```python
from build123d import *

# Parameters (mm, degrees)
SKETCH3_W                    = 914.4
SKETCH3_H                    = 609.6
BOSS_EXTRUDE1_DEPTH          = 0.79375
SKETCH4_OUTSIDE_W            = 1136.194
SKETCH4_OUTSIDE_H            = 831.394
CUT_EXTRUDE1_DEPTH           = 2.54
F_10_0_1935_DIAMETER_HOLE1_D = 4.9149
CUT_EXTRUDE5_DEPTH           = 2.54
CUT_EXTRUDE6_DEPTH           = 2.54
F_1_4_0_25_DIAMETER_HOLE1_D  = 6.35
F_10_CLEARANCE_HOLE1_D       = 4.9784


with BuildPart() as part:
    # Sketch3 → Boss-Extrude1 (new, symmetric)
    with BuildSketch(Plane.XY):
        Rectangle(SKETCH3_W, SKETCH3_H)
    extrude(amount=BOSS_EXTRUDE1_DEPTH, both=True)

    # Sketch4 outside → Cut-Extrude1 (cut)
    with BuildSketch(Plane.XY.offset(0.79375)):
        Rectangle(SKETCH4_OUTSIDE_W, SKETCH4_OUTSIDE_H)
        with BuildLine():
            Line((-362.506554298, 0.447439942), (318.21252852, 1.564886415))
            ThreePointArc((318.21252852, 1.564886415), (320.009798565, 0.823886977), (320.756694674, -0.970940586))
            Line((320.756694674, -0.970940586), (321.125317657, -225.526391983))
            Line((321.125317657, -225.526391983), (295.766909962, -250.884799679))
            Line((295.766909962, -250.884799679), (-339.232233443, -251.927193706))
            Line((-339.232233443, -251.927193706), (-364.674032102, -226.485395047))
            Line((-364.674032102, -226.485395047), (-365.0423813, -2.096726212))
            ThreePointArc((-365.0423813, -2.096726212), (-364.301381862, -0.299456167), (-362.506554298, 0.447439942))
        make_face(mode=Mode.SUBTRACT)
    extrude(amount=-CUT_EXTRUDE1_DEPTH, mode=Mode.SUBTRACT)

    # #10 (0.1935) Diameter Hole1 (through all)
    with Locations(Plane.XY.offset(0.79375)):
        with Locations((-301.153133674, -239.164667177), (-326.553099451, -239.206362941), (-351.97391311, -226.548075817), (-72.553441175, -238.789405326), (29.046421932, -238.622622281), (77.43654747, -240.486594059), (102.836513247, -240.444898294), (205.703184417, -238.332628273), (231.103150194, -238.290932508), (257.646113416, -238.247360435), (283.046079193, -238.205664671), (308.425197087, -225.463986018), (-155.475985843, -11.912722419), (111.223655321, -11.474916927)):
            Hole(F_10_0_1935_DIAMETER_HOLE1_D / 2)

    # Sketch13 → Cut-Extrude5 (cut)
    with BuildSketch(Plane(origin=(0, 0, -0.79375), x_dir=(-1, 0, 0), z_dir=(0, 0, -1))):
        with BuildLine():
            Line((-216.217386967, -166.841258451), (-343.254011981, -166.841258451))
            Line((-343.254011981, -166.841258451), (-342.941011359, 23.830509847))
            Line((-342.941011359, 23.830509847), (-152.613233115, 23.518073908))
            Line((-152.613233115, 23.518073908), (-152.613233115, -103.237104599))
            ThreePointArc((-152.613233115, -103.237104599), (-171.211866952, -148.242624615), (-216.217386967, -166.841258451))
        make_face()
    extrude(amount=-CUT_EXTRUDE5_DEPTH, mode=Mode.SUBTRACT)

    # Sketch12 → Cut-Extrude6 (cut)
    with BuildSketch(Plane(origin=(0, 0, -0.79375), x_dir=(-1, 0, 0), z_dir=(0, 0, -1))):
        with BuildLine():
            Line((196.636236426, -104.091867765), (196.636236426, 20.404753749))
            Line((196.636236426, 20.404753749), (384.763838571, 20.095930202))
            Line((384.763838571, 20.095930202), (384.455565363, -167.696021617))
            Line((384.455565363, -167.696021617), (260.031911457, -167.696021617))
            ThreePointArc((260.031911457, -167.696021617), (215.161222367, -149.023618888), (196.636236426, -104.091867765))
        make_face()
    extrude(amount=-CUT_EXTRUDE6_DEPTH, mode=Mode.SUBTRACT)

    # 1/4 (0.25) Diameter Hole1 (through all)
    with Locations(Plane(origin=(0, 0, -0.79375), x_dir=(-1, 0, 0), z_dir=(0, 0, -1))):
        with Locations((-142.973612542, -11.422797239), (187.225942556, -11.964842173)):
            Hole(F_1_4_0_25_DIAMETER_HOLE1_D / 2)

    # #10 Clearance Hole1 (through all)
    with Locations(Plane(origin=(0, 0, -0.79375), x_dir=(-1, 0, 0), z_dir=(0, 0, -1))):
        with Locations((-62.885205352, -101.186991996), (-19.917204705, -149.007237749), (46.027185416, -100.817324835), (106.973826127, -149.761638685)):
            Hole(F_10_CLEARANCE_HOLE1_D / 2)


solid = part.part
```
For this review, take the finished solid that the model builds, in its own axes (mm). Give positions to 0.01 mm unless a question says otherwise; leave off trailing zeros. Order: outer loops, then holes, each group sorted by start corner. A loop starts at its lowest first (then second) coordinate and runs counter-clockwise, first axis right, second up.
1) Wall thickness on line 1 (X direction, y = -171.5, z = -0.4); line 2 (Y direction, x = 27, z = -0.2); line 3 (X direction, y = -36.5, z = 0.45): over which ranges is each line inside the solid? List them lowest first.
2) Take a section at A-A (y = -43.5). Give the boundary of the cut face in (x, z), then the cut area to 3 significant figures.
3) Take a section at B-B (z = -0.5). State how many separate pieces and enclosed holes the cut face has, then the cut area to 3 significant figures.
4) Insertion check: pin 1 (10 mm diameter, centred on x = 142.97, y = -11.42, fed in from -Z). The pin has a flat end and moves straight along its axis. Give the tip position at first contact, or say it passes through.
5) Take a section at C-C (x = -227). Give the boundary of the cut face in (y, z), then the cut area to 3 significant figures.
Derived:
1. line 1: x = -364.76 to 321.04
1. line 2: y = -251.33 to -239.98, -237.26 to 1.09
1. line 3: x = -196.64 to 152.61
2. outline: (-196.64, -0.79) - (152.61, -0.79) - (152.61, 0.79) - (-196.64, 0.79) - close
2. area: 554 mm2
3. separate pieces: 1
3. enclosed holes: 20
3. area: 117,000 mm2
4. pin 1: stops at z = -0.79
5. outline: (-251.74, -0.79) - (-158.36, -0.79) - (-158.36, 0.79) - (-251.74, 0.79) - close
5. area: 148 mm2
